```python
from build123d import *

# Parameters (mm, degrees)
DODANIE_WYCI_GNI_CIE1_DEPTH = 10


with BuildPart() as part:
    # Szkic1 → Dodanie-wyciągnięcie1 (new body)
    with BuildSketch(Plane.XY):
        with BuildLine():
            Line((-327.852783983, -473.3081849), (-327.852783983, -478.408833405))
            Line((-327.852783983, -478.408833405), (-327.852783983, -479.408833405))
            ThreePointArc((-327.852783983, -479.408833405), (-326.974104327, -481.530153749), (-324.852783983, -482.408833405))
            Line((-324.852783983, -482.408833405), (-320.102783983, -482.408833405))
            Line((-320.102783983, -482.408833405), (-311.752783983, -482.408833405))
            ThreePointArc((-311.752783983, -482.408833405), (-310.338570421, -481.823046968), (-309.752783983, -480.408833405))
            Line((-309.752783983, -480.408833405), (-309.752783983, -472.318864182))
            Line((-309.752783983, -472.318864182), (-300.552783983, -472.318864182))
            Line((-300.552783983, -472.318864182), (-289.552783983, -472.318864182))
            Line((-289.552783983, -472.318864182), (-289.552783983, -477.218864182))
            Line((-289.552783983, -477.218864182), (-294.252783983, -477.218864182))
            Line((-294.252783983, -477.218864182), (-294.252783983, -475.843864182))
            Line((-294.252783983, -475.843864182), (-296.252783983, -475.843864182))
            Line((-296.252783983, -475.843864182), (-296.252783983, -477.218864182))
            Line((-296.252783983, -477.218864182), (-296.752783983, -477.218864182))
            Line((-296.752783983, -477.218864182), (-296.752783983, -480.318864182))
            Line((-296.752783983, -480.318864182), (-296.252783983, -480.318864182))
            Line((-296.252783983, -480.318864182), (-296.252783983, -481.693864182))
            Line((-296.252783983, -481.693864182), (-294.252783983, -481.693864182))
            Line((-294.252783983, -481.693864182), (-294.252783983, -480.318864182))
            Line((-294.252783983, -480.318864182), (-289.552783983, -480.318864182))
            Line((-289.552783983, -480.318864182), (-289.552783983, -484.318864182))
            Line((-289.552783983, -484.318864182), (-283.552783983, -484.318864182))
            Line((-283.552783983, -484.318864182), (-283.552783983, -490.318864182))
            Line((-283.552783983, -490.318864182), (-289.552783983, -490.318864182))
            Line((-289.552783983, -490.318864182), (-289.552783983, -494.315935469))
            Line((-289.552783983, -494.315935469), (-289.552783983, -500.21329504))
            Line((-289.552783983, -500.21329504), (-327.723397777, -491.496448064))
            ThreePointArc((-327.723397777, -491.496448064), (-331.658671111, -489.587789306), (-333.252783983, -485.514932984))
            Line((-333.252783983, -485.514932984), (-333.252783983, -470.917158488))
            ThreePointArc((-333.252783983, -470.917158488), (-330.552783983, -471.708833405), (-327.852783983, -470.917158488))
            Line((-327.852783983, -470.917158488), (-327.852783983, -473.3081849))
        make_face()
    extrude(amount=DODANIE_WYCI_GNI_CIE1_DEPTH)


solid = part.part
```
The listing builds one solid part. Answer for the finished solid, in the listing's coordinates (mm). A direction names the side the tool comes from. Round coordinates to 2 decimals unless told otherwise and drop trailing zeros. Write each loop counter-clockwise with the first axis right and the second up, starting at its lowest first coordinate (ties: lowest second). Pieces come first, ordered by that corner, then holes. Notation, with made-up numbers: (52, 31) -> (90, 31) arc R16 ccw to (90, 43) -> close; hole circle Ø9 at (48.25, 25). An arc over 180 degrees is marked (long way). Use CSV: the item, a comma, the result in double quotes. Start each with the question number.
(1) Section C-C on y = -483.5 is taken. Give the vertices of the cut face in (x, z).
(2) Section B-B on x = -291 is taken. Give the vertices of the cut face in (y, z).
(3) Which of the six approach directions +Z, -Z, +X, -X, +Y, -Y give full straight-line access (tool end or side, diameter ignored) to faces 4 (the face through (-292, -480.319, 5)), 5 (the face through (-296.253, -477, 5)), 6 (the face through (-300, -472.319, 5))?
(4) Consider L1, parallel to X at y = -477.5, z = 1.5; L2, parallel to X at y = -480.5, z = 3.75; L3, parallel to Y at x = -287.5, z = 1. Determine where each line is inside the solid, lowest interval first. Write a range as from..to.
(5) Section D-D on x = -326 is taken. Give the vertices of the cut face in (y, z), then the cut area to 3 significant figures.
(6) Section A-A on z = 4.5 is taken. Give the vertices of the cut face in (x, y), then the cut area to 3 significant figures.
(7) Each of these flat-tipped pins is pushed along its axis until it touches: pin 1 (3 mm diameter, centred on y = -482, z = 2.5, fed in from +X); pin 2 (4 mm diameter, centred on x = -309.5, z = 6.5, fed in from +Y); pin 3 (1.8 mm diameter, centred on x = -285.5, z = 4.5, fed in from +Y). Where does it stop, or does it pass through?
(8) The mould has two halves that part along Y. Classify faces 1 (the face through (-327.853, -475, 5)), 2 (the face through (-310.354, -481.839, 4.93)), 3 (the face through (-295, -481.694, 5)): released by +Y, released by -Y, zero draft, split by the parting line, or undercut.
A:
1,outline,"(-333.25, 0) -> (-289.55, 0) -> (-289.55, 10) -> (-333.25, 10) -> close"
2,outline,"(-499.88, 0) -> (-480.32, 0) -> (-480.32, 10) -> (-499.88, 10) -> close; (-477.22, 0) -> (-472.32, 0) -> (-472.32, 10) -> (-477.22, 10) -> close"
3,face 4,"+Z, -Z, +X"
3,face 5,"+Z, -Z"
3,face 6,"+Z, -Z, +X, +Y"
4,L1,"x = -333.25..-327.85, -309.75..-296.75"
4,L2,"x = -333.25..-327.65, -309.75..-296.25, -294.25..-289.55"
4,L3,"y = -490.32..-484.32"
5,outline,"(-491.89, 0) -> (-482.18, 0) -> (-482.18, 10) -> (-491.89, 10) -> close"
5,area,"97.1 mm²"
6,outline,"(-333.25, -485.51) arc R6 ccw to (-327.72, -491.5) -> (-289.55, -500.21) -> (-289.55, -490.32) -> (-283.55, -490.32) -> (-283.55, -484.32) -> (-289.55, -484.32) -> (-289.55, -480.32) -> (-294.25, -480.32) -> (-294.25, -481.69) -> (-296.25, -481.69) -> (-296.25, -480.32) -> (-296.75, -480.32) -> (-296.75, -477.22) -> (-296.25, -477.22) -> (-296.25, -475.84) -> (-294.25, -475.84) -> (-294.25, -477.22) -> (-289.55, -477.22) -> (-289.55, -472.32) -> (-309.75, -472.32) -> (-309.75, -480.41) arc R2 cw to (-311.75, -482.41) -> (-324.85, -482.41) arc R3 cw to (-327.85, -479.41) -> (-327.85, -470.92) arc R5 cw to (-333.25, -470.92) -> close"
6,area,"830 mm²"
7,pin 1,"stops at x = -289.55"
7,pin 2,"stops at y = -472.32"
7,pin 3,"stops at y = -484.32"
8,face 1,"zero draft"
8,face 2,"released by +Y"
8,face 3,"undercut"
